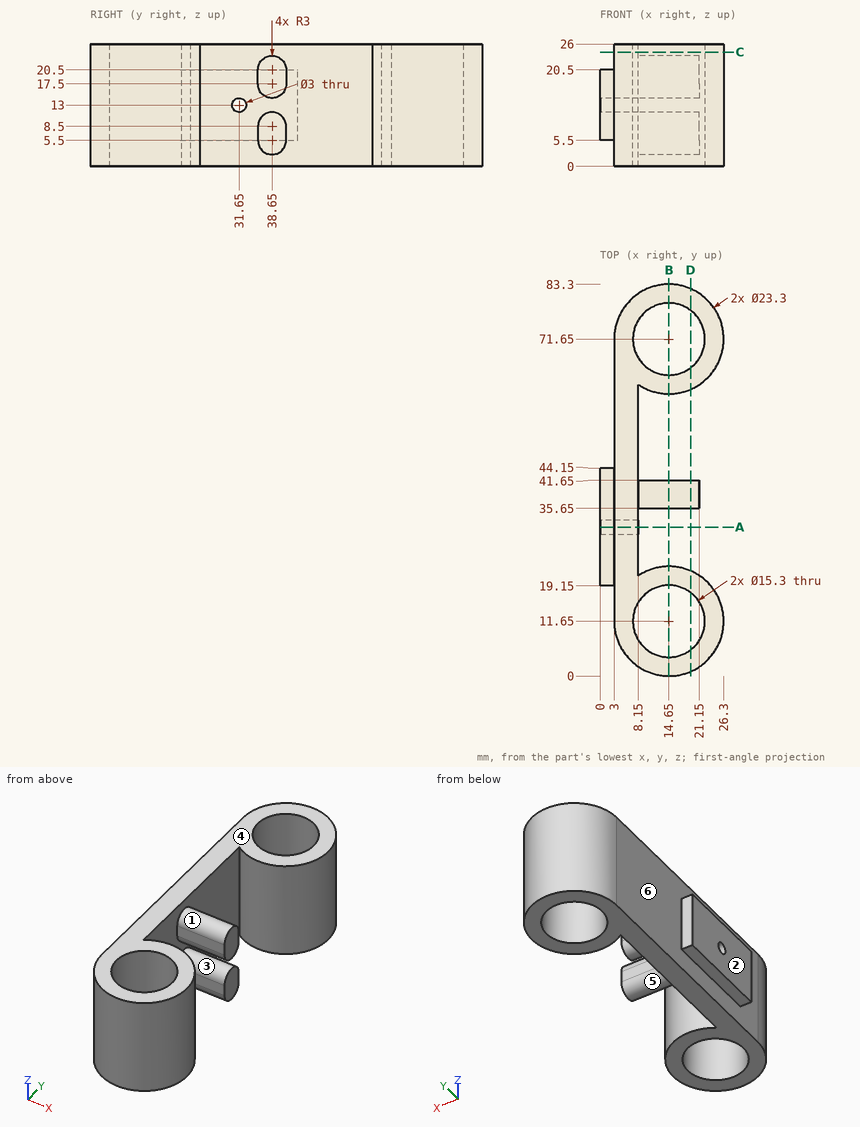
Answer from the drawing. Dimensions are ordinates in mm from the lowest x, y and z of the part. A direction names the side the tool comes from. Round coordinates to 2 decimals unless told otherwise and drop trailing zeros. Loops run counter-clockwise (first coordinate to the right, second up) from the corner with the lowest first, then second, coordinate; pieces in that order, holes last. Notation, with made-up numbers: (41, -5.5) - (66, -5.5) arc R31 cw to (66, 19.5) - close; hole circle Ø7 at (37.5, 71.5). An arc over 180 degrees is marked (long way). One line per item, written item: value.
Q1. Each of these flat-tipped pins is pushed along its axis until it touches: pin 1 Ø0.9 at (x, y) = (2, 34.5) entering from +Z; pin 2 Ø4 at (y, z) = (16, 9) entering from +X; pin 3 Ø0.9 at (x, y) = (1.5, 38) entering from -Z. Where does it stop, or does it pass through?
Check values:
pin 1: z = 20.5
pin 2: x = 26.06
pin 3: z = 5.5
Q2. Find section A-A on y = 31.65. Give the vertices of the cut face in (x, z), and give its area (3 significant figures).
Check values:
outline: (0, 5.5) - (3, 5.5) - (3, 0) - (8.15, 0) - (8.15, 11.5) - (0, 11.5) - close; (0, 14.5) - (8.15, 14.5) - (8.15, 26) - (3, 26) - (3, 20.5) - (0, 20.5) - close
area: 154 mm2
Q3. Find section C-C on z = 24.25. Give the vertices of the cut face in (x, y), and give its area (3 significant figures).
Check values:
outline: (3, 11.65) arc R11.65 ccw (long way) to (8.15, 21.32) - (8.15, 61.98) arc R11.65 ccw (long way) to (3, 71.65) - close; hole circle Ø15.3 at (14.65, 11.65); hole circle Ø15.3 at (14.65, 71.65)
area: 724 mm2
Q4. Straight lines are drawn through the part: probe 1 along Y at (x, z) = (14.25, 12); probe 2 along Z at (x, y) = (1.5, 31.65); probe 3 along Y at (x, z) = (17.75, 21.5). For each, find the intervals that lie inside material, in ascending order.
Check values:
probe 1: 0.01 to 4.01, 19.29 to 23.29, 60.01 to 64.01, 79.29 to 83.29
probe 2: 5.5 to 11.5, 14.5 to 20.5
probe 3: 0.42 to 4.66, 18.64 to 22.88, 35.82 to 41.48, 60.42 to 64.66, 78.64 to 82.88
Q5. Find section D-D on x = 19.25. Give the vertices of the cut face in (y, z).
Check values:
outline: (0.95, 0) - (5.54, 0) - (5.54, 26) - (0.95, 26) - close; (17.76, 0) - (22.35, 0) - (22.35, 26) - (17.76, 26) - close; (35.65, 5.5) arc R3 ccw to (41.65, 5.5) - (41.65, 8.5) arc R3 ccw to (35.65, 8.5) - close; (35.65, 17.5) arc R3 ccw to (41.65, 17.5) - (41.65, 20.5) arc R3 ccw to (35.65, 20.5) - close; (60.95, 0) - (65.54, 0) - (65.54, 26) - (60.95, 26) - close; (77.76, 0) - (82.35, 0) - (82.35, 26) - (77.76, 26) - close
Q6. For the marked faces 1 and 2, determine the directions among +Z, -Z, +X, -X, +Y, -Y from which every point of the face is accessible in a straight line to the end or side of a thin tool.
Check values:
face 1: +Z, +X
face 2: +Z, -Z, -X, +Y, -Y
Q7. Find section B-B on x = 14.65. Give the vertices of the cut face in (y, z), and give its area (3 significant figures).
Check values:
outline: (0, 0) - (4, 0) - (4, 26) - (0, 26) - close; (19.3, 0) - (23.3, 0) - (23.3, 26) - (19.3, 26) - close; (35.65, 5.5) arc R3 ccw to (41.65, 5.5) - (41.65, 8.5) arc R3 ccw to (35.65, 8.5) - close; (35.65, 17.5) arc R3 ccw to (41.65, 17.5) - (41.65, 20.5) arc R3 ccw to (35.65, 20.5) - close; (60, 0) - (64, 0) - (64, 26) - (60, 26) - close; (79.3, 0) - (83.3, 0) - (83.3, 26) - (79.3, 26) - close
area: 509 mm2
Q8. The mould has two halves that part along Z. Classify the marked faces 3, 4, 5 and 6: +Z half, -Z half, draft (parallel to the pull), parting line (faces both ways), or undercut.
Check values:
face 3: undercut
face 4: +Z half
face 5: -Z half
face 6: draft
